Input: part model. Units: mm. Frame: model coordinates. Give positions to 0.01 mm unless a question says otherwise; leave off trailing zeros. Write each loop counter-clockwise with the first axis right and the second up, starting at its lowest first coordinate (ties: lowest second). Pieces come first, ordered by that corner, then holes. Notation, with made-up numbers: (-12, 23) -> (44, 23) arc R15 ccw to (44, 35) -> close; hole circle Ø11 at (72, 89.25). An arc over 180 degrees is marked (long way). Answer as a JSON object with one key per item and string values. Group by question number.
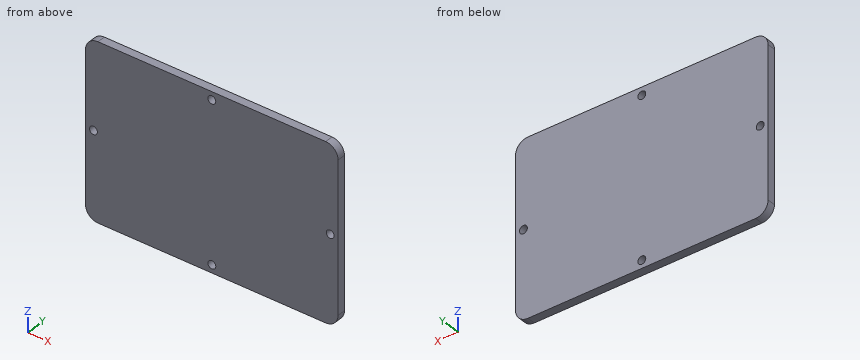
from build123d import *

# Parameters (mm, degrees)
SKETCH1_W           = 101.6
SKETCH1_H           = 69.85
BOSS_EXTRUDE1_DEPTH = 3.302
SKETCH4_R           = 1.5875
CUT_EXTRUDE1_DEPTH  = 4.302
FILLET1_R           = 5


with BuildPart() as part:
    # Sketch1 → Boss-Extrude1 (new body)
    with BuildSketch(Plane(origin=(0, 0, 0), x_dir=(1, 0, 0), z_dir=(0, 1, 0))):
        Rectangle(SKETCH1_W, SKETCH1_H)
    extrude(amount=BOSS_EXTRUDE1_DEPTH)

    # Sketch4 → Cut-Extrude1 (cut, through all)
    with BuildSketch(Plane(origin=(0, 0, 0), x_dir=(-1, 0, 0), z_dir=(0, -1, 0))):
        with Locations((0, 31.75)):
            Circle(SKETCH4_R)
        with Locations((-47.625, 0)):
            Circle(SKETCH4_R)
        with Locations((0, -31.75)):
            Circle(SKETCH4_R)
        with Locations((47.625, 0)):
            Circle(SKETCH4_R)
    extrude(amount=-CUT_EXTRUDE1_DEPTH, mode=Mode.SUBTRACT)

    # Fillet1
    fillet1_edges = [part.edges().sort_by_distance(p)[0] for p in [
        (50.8, 1.651, 34.925),
        (-50.8, 1.651, 34.925),
        (-50.8, 1.651, -34.925),
        (50.8, 1.651, -34.925),
    ]]
    fillet(fillet1_edges, radius=FILLET1_R)


solid = part.part
1. Section C-C (z = 31.75). Return the cut outline in (x, y), plus the area to 3 significant figures.
2. Line query: line 1 (X direction, y = 1.7, z = 0); line 2 (Z direction, x = 0, y = 1.7) (1 decimal); line 3 (X direction, y = 2.4, z = -31.75). Output: solid intervals per line, ascending.
3. Section A-A (x = 0). Return the cut outline in (y, z) (1 decimal), plus the area to 3 significant figures.
4. Section B-B (z = 0). Return the cut outline in (x, y), plus the area to 3 significant figures.
Working result:
{
 "1": {"outline": "(-50.46, 0) -> (-1.59, 0) -> (-1.59, 3.3) -> (-50.46, 3.3) -> close; (1.59, 0) -> (50.46, 0) -> (50.46, 3.3) -> (1.59, 3.3) -> close", "area": "323 mm^2"},
 "2": {"line 1": "x = -50.8 to -49.21, -46.04 to 46.04, 49.21 to 50.8", "line 2": "z = -34.9 to -33.3, -30.2 to 30.2, 33.3 to 34.9", "line 3": "x = -50.46 to -1.59, 1.59 to 50.46"},
 "3": {"outline": "(0, -34.9) -> (3.3, -34.9) -> (3.3, -33.3) -> (0, -33.3) -> close; (0, -30.2) -> (3.3, -30.2) -> (3.3, 30.2) -> (0, 30.2) -> close; (0, 33.3) -> (3.3, 33.3) -> (3.3, 34.9) -> (0, 34.9) -> close", "area": "210 mm^2"},
 "4": {"outline": "(-50.8, 0) -> (-49.21, 0) -> (-49.21, 3.3) -> (-50.8, 3.3) -> close; (-46.04, 0) -> (46.04, 0) -> (46.04, 3.3) -> (-46.04, 3.3) -> close; (49.21, 0) -> (50.8, 0) -> (50.8, 3.3) -> (49.21, 3.3) -> close", "area": "315 mm^2"}
}
